Input: part model. Units: mm. Frame: model coordinates. Face numbers are marked on the shaded views. A direction names the side the tool comes from. Coordinates: 2 decimals unless noted, no trailing zeros. Write each loop counter-clockwise with the first axis right and the second up, starting at its lowest first coordinate (ties: lowest second). Pieces come first, ordered by that corner, then holes. Notation, with made-up numbers: M 31,-12.5 L 78,-12.5 A31 cw 78,18.5 Z; hole C 26,75.5 d6. An arc over 180 degrees is marked long. Use one line per item in the form item = value.
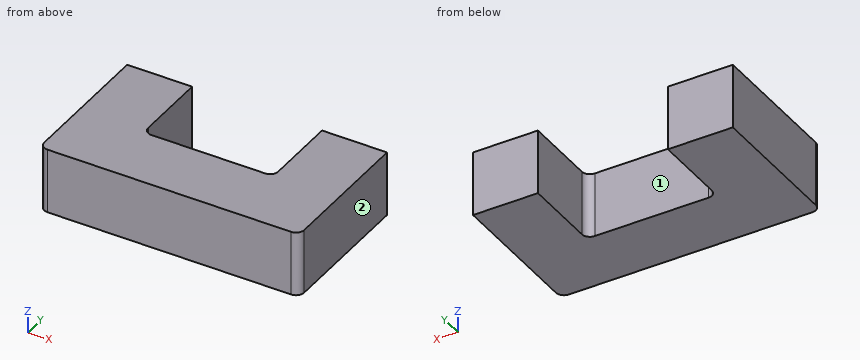
Autodesk Inventor part; units mm, degrees
ref_plane "YZ Plane" through (0, 0, 0) normal (1, 0, 0) x (0, 1, 0)
ref_plane "XZ Plane" through (0, 0, 0) normal (0, 1, 0) x (-1, 0, 0)
ref_plane "XY Plane" through (0, 0, 0) normal (0, 0, 1) x (1, 0, 0)
sketch "Sketch1" plane through (0, 0, 0) normal (0, 0, 1) x (1, 0, 0)
  line L0 (-21.2406, 0) -> (122.8406, 0)
  line L1 (0, -12.2191) -> (0, 68.7115)
  line L2 (3.175, 0) -> (98.425, 0)
  line L3 (101.6, 3.175) -> (101.6, 25.4)
  line L4 (73.025, 25.4) -> (28.575, 25.4)
  line L5 (0, 25.4) -> (0, 3.175)
  line L6 (0, 25.4) -> (25.4, 25.4)
  line L7 (25.4, 28.575) -> (25.4, 57.15)
  line L8 (25.4, 57.15) -> (0, 57.15)
  line L9 (0, 57.15) -> (0, 25.4)
  line L10 (76.2, 57.15) -> (101.6, 57.15)
  line L11 (101.6, 57.15) -> (101.6, 25.4)
  line L12 (101.6, 25.4) -> (76.2, 25.4)
  line L13 (76.2, 28.575) -> (76.2, 57.15)
  arc A0 (25.4, 28.575) -> (28.575, 25.4) centre (28.575, 28.575) ccw
  arc A1 (73.025, 25.4) -> (76.2, 28.575) centre (73.025, 28.575) ccw
  arc A2 (98.425, 0) -> (101.6, 3.175) centre (98.425, 3.175) ccw
  arc A3 (0, 3.175) -> (3.175, 0) centre (3.175, 3.175) ccw
  point P0 (0, 0)
  point P1 (101.6, 0)
  dimension "d0" = 101.6
  dimension "d1" = 25.4
  dimension "d2" = 25.4
  dimension "d3" = 57.15
  dimension "d4" = 25.4
  dimension "d5" = 57.15
  dimension "d6" = 3.175
extrude "Extrusion1" add sketch "Sketch1" along normal blind 25.4 contours A3 L1 L8 L7 A0 L4 A1 L13 L10 L11 L3 A2 L0
properties part number "ferrite_core"
(1) First-contact query: pin 1 Ø1.5 at (x, z) = (51, 13) entering from +Y; pin 2 Ø1 at (x, y) = (86.5, 45.5) entering from -Z; pin 3 Ø1 at (x, z) = (28, 11.5) entering from +Y. Flat tips, straight axial feed; report the tip coordinate or a pass-through.
Computed:
pin_1 = 25.4
pin_2 = 0
pin_3 = 25.59
(2) Section query A-A on y = 42. Return the cut outline in (x, z).
Computed:
outline = M 0,0 L 25.4,0 L 25.4,25.4 L 0,25.4 Z; M 76.2,0 L 101.6,0 L 101.6,25.4 L 76.2,25.4 Z
(3) Section query C-C on x = 53.5. Return the cut outline in (y, z), plus the area to 3 significant figures.
Computed:
outline = M 0,0 L 25.4,0 L 25.4,25.4 L 0,25.4 Z
area = 645 mm^2
(4) Set-up query: the marked faces 1 and 2. Return all of +Z, -Z, +X, -X, +Y, -Y with unobstructed straight access to the full face (end or side cutting, diameter ignored); none if empty.
Computed:
face_1 = +Z, -Z, +Y
face_2 = +Z, -Z, +X, +Y, -Y
(5) Line query: probe 1 along X at (y, z) = (49.5, 9.25); probe 2 along Y at (x, z) = (45, 9.25); probe 3 along X at (y, z) = (27, 17.25). Output: solid intervals per line, ascending.
Computed:
probe_1 = 0 to 25.4, 76.2 to 101.6
probe_2 = 0 to 25.4
probe_3 = 0 to 25.82, 75.78 to 101.6
(6) Section query D-D on x = 27. Return the cut outline in (y, z), plus the area to 3 significant figures.
Computed:
outline = M 0,0 L 25.82,0 L 25.82,25.4 L 0,25.4 Z
area = 656 mm^2
(7) Section query B-B on z = 13.5. Return the cut outline in (x, y) (3 decimals).
Computed:
outline = M 0,3.175 A3.175 ccw 3.175,0 L 98.425,0 A3.175 ccw 101.6,3.175 L 101.6,57.15 L 76.2,57.15 L 76.2,28.575 A3.175 cw 73.025,25.4 L 28.575,25.4 A3.175 cw 25.4,28.575 L 25.4,57.15 L 0,57.15 Z
